Can you work these out from the model? Positions are in its coordinate system, mm. Face numbers are marked on the shaded views. A direction names the side the tool comes from. Round coordinates to 2 decimals unless told otherwise and drop trailing zeros. Write each loop counter-clockwise with the first axis right and the second up, starting at its lowest first coordinate (ties: lowest second). Pieces come first, ordered by that corner, then holes. Notation, with made-up numbers: M 66,-1.5 L 72,-1.5 A17 cw 72,10.5 Z; hole C 58.25,69 d1. An arc over 180 degrees is marked long. Answer as a JSON object with one key per item and string values. Group by question number.
1) I'm going to push flat-ended pins straight in: pin 1 Ø12 at (x, z) = (36, 20) entering from -Y; pin 2 Ø4 at (x, y) = (25, 94.59) entering from +Z; pin 3 Ø10 at (x, z) = (16, 38.5) entering from +Y. Where does each tip first touch, or does it pass through?
2) If we mould it in two halves opening along Z, with no side actions, what happens to the marked faces 1, 2, 3 and 4? For each: +Z half, -Z half, draft (parallel to the pull), parting line (faces both ways), or undercut.
3) Please list where these lines run through material, in increasing order: L1, parallel to Z at x = 44, y = 35.5; L2, parallel to Y at x = 25, z = 7; L3, parallel to X at y = 66, z = 33. Write a range as [from, to].
4) Suppose I cut it at C-C, the plane z = 30. Write out the boundary of the cut face in (x, y).
5) On a 3-axis mill with a long thin cutter (end or side, diameter ignored), from which of +Z, -Z, +X, -X, +Y, -Y can I reach the whole of each face in a straight line? I mean the marked faces 5 and 6. Say none if no direction works.
6) Suppose I cut it at B-B, the plane x = 16. Write out the boundary of the cut face in (y, z), and give its area (3 significant figures).
7) Suppose I cut it at A-A, the plane y = 47.5. Write out the boundary of the cut face in (x, z), and give its area (3 significant figures).
8) Suppose I cut it at D-D, the plane y = 71.5. Write out the boundary of the cut face in (x, z), and give its area (3 significant figures).
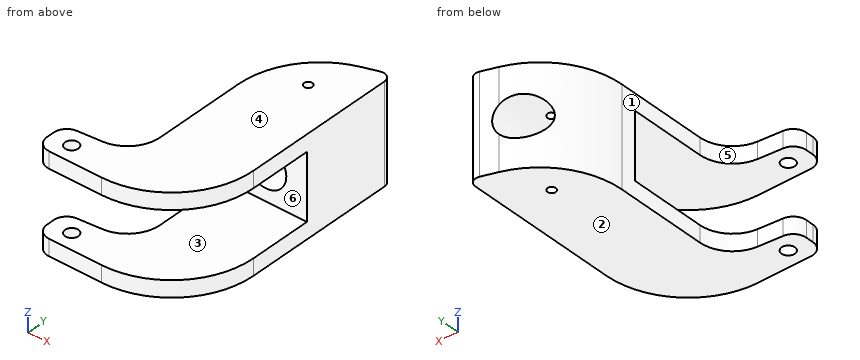
from build123d import *

# Parameters (mm, degrees)
SKETCH1_R               = 4
BOSS_EXTRUDE1_DEPTH     = 60
CUT_EXTRUDE1_DEPTH      = 148.042397089
CUT_EXTRUDE1_DEPTH_BACK = 148.042397089
SKETCH2_W               = 40
SKETCH2_H               = 100
CUT_EXTRUDE2_DEPTH      = 148.042397089
CUT_EXTRUDE2_DEPTH_BACK = 148.042397089
SKETCH4_R               = 12.5
CUT_EXTRUDE3_DEPTH      = 148.04239713
CUT_EXTRUDE3_DEPTH_BACK = 148.04239713
SKETCH5_R               = 2.5


with BuildPart() as part:
    # Sketch1 → Boss-Extrude1 (new body)
    with BuildSketch(Plane.XY):
        with BuildLine():
            Line((0, 18.32662348), (0, 73.848150904))
            ThreePointArc((0, 73.848150904), (9.481713685, 103.144370354), (34.330738963, 121.329455209))
            Line((34.330738963, 121.329455209), (43.433073896, 124.333308288))
            ThreePointArc((43.433073896, 124.333308288), (47.929621945, 123.637006489), (50, 119.585177858))
            Line((50, 119.585177858), (50, 26.500453459))
            ThreePointArc((50, 26.500453459), (35.355339059, -8.8548856), (0, -23.499546541))
            Line((0, -23.499546541), (-32, -23.499546541))
            ThreePointArc((-32, -23.499546541), (-37.656854249, -21.156400791), (-40, -15.499546541))
            Line((-40, -15.499546541), (-40, -10.830195933))
            ThreePointArc((-40, -10.830195933), (-37.898218694, -5.425474272), (-32.697245942, -2.860638348))
            Line((-32.697245942, -2.860638348), (-18.256885145, -1.597270481))
            ThreePointArc((-18.256885145, -1.597270481), (-5.254453264, 4.814819328), (0, 18.32662348))
        make_face()
        with Locations((-27, -13.164871237)):
            Circle(SKETCH1_R, mode=Mode.SUBTRACT)
    extrude(amount=BOSS_EXTRUDE1_DEPTH)

    # Sketch2 → Cut-Extrude1 (cut, two sides: drawn at the far end of the back side and taken through both)
    with BuildSketch(Plane(origin=(0, 0, 0), x_dir=(0, 0, -1), z_dir=(1, 0, 0)).offset(-CUT_EXTRUDE1_DEPTH_BACK)):
        with Locations((-30, 14.333308288)):
            Rectangle(SKETCH2_W, SKETCH2_H)
    extrude(amount=CUT_EXTRUDE1_DEPTH + CUT_EXTRUDE1_DEPTH_BACK, mode=Mode.SUBTRACT)

    # Sketch4 → Cut-Extrude2 (cut, two sides: drawn at the far end of the back side and taken through both)
    with BuildSketch(Plane(origin=(0, 0, 0), x_dir=(1, 0, 0), z_dir=(0, 1, 0)).offset(-CUT_EXTRUDE2_DEPTH_BACK)):
        with Locations(Location((25, -30, 0), (0, 0, 270))):
            Circle(SKETCH4_R)
    extrude(amount=CUT_EXTRUDE2_DEPTH + CUT_EXTRUDE2_DEPTH_BACK, mode=Mode.SUBTRACT)

    # Sketch5 → Cut-Extrude3 (cut, two sides: drawn at the far end of the back side and taken through both)
    with BuildSketch(Plane.XY.offset(60).offset(-CUT_EXTRUDE3_DEPTH_BACK)):
        with Locations((25, 94.585177858)):
            Circle(SKETCH5_R)
    extrude(amount=CUT_EXTRUDE3_DEPTH + CUT_EXTRUDE3_DEPTH_BACK, mode=Mode.SUBTRACT)


solid = part.part
Results:
{
 "1": {"pin 1": "y = 64.33", "pin 2": "through", "pin 3": "y = 113.87"},
 "2": {"face 1": "draft", "face 2": "-Z half", "face 3": "undercut", "face 4": "+Z half"},
 "3": {"L1": "[0, 10], [50, 60]", "L2": "[-16.8, 92.09], [97.09, 117.15]", "L3": "[0, 12.87], [37.13, 50]"},
 "4": {"outline": "M 0,64.33 L 12.5,64.33 L 12.5,106.92 A50 ccw 0,73.85 Z; M 37.5,64.33 L 50,64.33 L 50,119.59 A5 ccw 43.43,124.33 L 37.5,122.38 Z"},
 "5": {"face 5": "+Z, -Z, -X, +Y", "face 6": "+X, -X, -Y"},
 "6": {"outline": "M -20.87,0 L 110.51,0 L 110.51,21.33 L 64.33,21.33 L 64.33,10 L -20.87,10 Z; M -20.87,50 L 64.33,50 L 64.33,38.67 L 110.51,38.67 L 110.51,60 L -20.87,60 Z", "area": "3,670 mm^2"},
 "7": {"outline": "M 0,0 L 50,0 L 50,10 L 0,10 Z; M 0,50 L 50,50 L 50,60 L 0,60 Z", "area": "1,000 mm^2"},
 "8": {"outline": "M 0,0 L 50,0 L 50,60 L 0,60 Z; hole C 25,30 d25", "area": "2,510 mm^2"}
}
